from build123d import *

# Parameters (mm, degrees)
SKETCH_1_R      = 22
EXTRUDE_1_DEPTH = 14
SKETCH_2_R      = 32
EXTRUDE_2_DEPTH = 10
SKETCH_3_W      = 56
SKETCH_3_H      = 74
EXTRUDE_3_DEPTH = 24
SKETCH_4_W      = 6
SKETCH_4_H      = 74
EXTRUDE_4_DEPTH = 76


with BuildPart() as part:
    # 草图1 → 凸台-拉伸1 (new body)
    with BuildSketch(Plane.XY):
        Circle(SKETCH_1_R)
    extrude(amount=-EXTRUDE_1_DEPTH)

    # 草图2 → 凸台-拉伸2 (add)
    with BuildSketch(Plane.XY):
        Circle(SKETCH_2_R)
    extrude(amount=EXTRUDE_2_DEPTH)

    # 草图3 → 凸台-拉伸3 (add)
    with BuildSketch(Plane.XY):
        Rectangle(SKETCH_3_W, SKETCH_3_H)
    extrude(amount=EXTRUDE_3_DEPTH)

    # 草图4 → 凸台-拉伸4 (add)
    with BuildSketch(Plane.XY):
        with Locations((23, 0)):
            Rectangle(SKETCH_4_W, SKETCH_4_H)
        with Locations((-23, 0)):
            Rectangle(SKETCH_4_W, SKETCH_4_H)
    extrude(amount=EXTRUDE_4_DEPTH)


solid = part.part
Could you check a few things on this model? Use its own coordinates, in mm. A direction names the side the tool comes from. Give positions to 0.01 mm unless a question says otherwise; leave off trailing zeros. Order: outer loops, then holes, each group sorted by start corner. A loop starts at its lowest first (then second) coordinate and runs counter-clockwise, first axis right, second up. Notation, with made-up numbers: (-32, 54) - (9, 54) arc R26 ccw to (9, 78) - close; hole circle Ø6 at (12, 53.25). An arc over 180 degrees is marked (long way). One line per item, written item: value. Start each with the question number.
1. Imagine slicing it at A-A on z = 28. List the corners of the cut face in (x, y) for me.
2. If I drill on probe 1 along X at (y, z) = (13.5, 52); probe 2 along Z at (x, y) = (-11, 24); probe 3 along X at (y, z) = (13.5, 14), over which ranges is the centre line in solid material (lowest first)?
3. Imagine slicing it at B-B on x = 0. List the corners of the cut face in (y, z) for me, plus the area to 3 significant figures.
4. For faces 1 (the face through (-28, -1, 12)), 2 (the face through (-30, 0, 10)), 3 (the face through (28, -1, 12)), 4 (the face through (21, 9, 0)), which set-ups out of +Z, -Z, +X, -X, +Y, -Y let a thin tool reach every point of the face, with its end or its side?
5. Imagine slicing it at C-C on y = 0. List the corners of the cut face in (x, z) for me, plus the area to 3 significant figures.
6. Imagine slicing it at D-D on z = 7. List the corners of the cut face in (x, y) for me.
7. For P1, Ø20, axis at x = 6, y = -15.5, coming from the +Z side; P2, Ø19, axis at y = -11.5, z = 8.5, coming from the -X side; P3, Ø3, axis at x = 30, y = 3.5, coming from the +Z side; P4, Ø12, axis at x = 25.5, y = -8, coming from the -Z side, each with a flat end and sliding along its axis, tell me the tip position at first contact or that it passes through.
Values:
1. outline: (-26, -37) - (-20, -37) - (-20, 37) - (-26, 37) - close; (20, -37) - (26, -37) - (26, 37) - (20, 37) - close
2. probe 1: -26 to -20, 20 to 26
2. probe 2: 0 to 24
2. probe 3: -28 to 28
3. outline: (-37, 0) - (-22, 0) - (-22, -14) - (22, -14) - (22, 0) - (37, 0) - (37, 24) - (-37, 24) - close
3. area: 2,390 mm²
4. face 1: +Z, -X
4. face 2: +Z, -X, +Y, -Y
4. face 3: +Z, +X
4. face 4: -Z
5. outline: (-32, 0) - (-22, 0) - (-22, -14) - (22, -14) - (22, 0) - (32, 0) - (32, 10) - (28, 10) - (28, 24) - (26, 24) - (26, 76) - (20, 76) - (20, 24) - (-20, 24) - (-20, 76) - (-26, 76) - (-26, 24) - (-28, 24) - (-28, 10) - (-32, 10) - close
5. area: 2,660 mm²
6. outline: (-28, -37) - (28, -37) - (28, -15.49) arc R32 ccw to (28, 15.49) - (28, 37) - (-28, 37) - (-28, 15.49) arc R32 ccw to (-28, -15.49) - close
7. P1: z = 24
7. P2: x = -31.94
7. P3: z = 10
7. P4: z = -14
